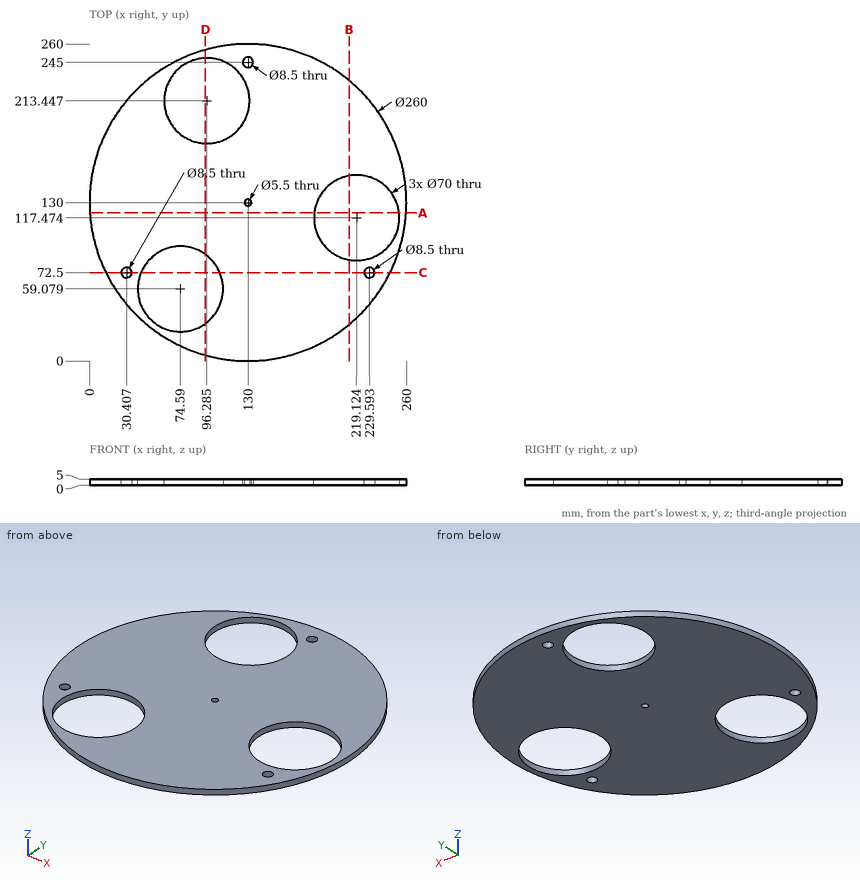
Drawing for the job (mm, zero at the part's lowest x, y, z). Round coordinates to 2 decimals unless told otherwise and drop trailing zeros. Write each loop counter-clockwise with the first axis right and the second up, starting at its lowest first coordinate (ties: lowest second). Pieces come first, ordered by that corner, then holes. Notation, with made-up numbers: M 66.5,-14.5 L 108.5,-14.5 A18 cw 108.5,-9.5 Z; hole C 5.5,47 d8. An arc over 180 degrees is marked long. Answer in a Markdown table with one row per item.
1. Saw through at A-A (y = 121.5). List the corners of the cut face in (x, z).
Geometry check:
| item | result |
|---|---|
| outline | M 0.28,0 L 184.36,0 L 184.36,5 L 0.28,5 Z; M 253.89,0 L 259.72,0 L 259.72,5 L 253.89,5 Z |
2. Saw through at D-D (x = 95). List the corners of the cut face in (y, z) (1 decimal).
Geometry check:
| item | result |
|---|---|
| outline | M 4.8,0 L 30.6,0 L 30.6,5 L 4.8,5 Z; M 87.5,0 L 178.5,0 L 178.5,5 L 87.5,5 Z; M 248.4,0 L 255.2,0 L 255.2,5 L 248.4,5 Z |
3. Probe L1, parallel to Y at x = 97, z = 2.85 (1 decimal); L2, parallel to X at y = 128, z = 2.9 (1 decimal); L3, parallel to Y at x = 69, z = 4.7 (1 decimal). List the from-to ranges inside material, lowest first. Write a range as [from, to].
Geometry check:
| item | result |
|---|---|
| L1 | [4.3, 32.2], [86, 178.5], [248.4, 255.7] |
| L2 | [0, 128.1], [131.9, 185.7], [252.5, 260] |
| L3 | [15.2, 24.5], [93.6, 191.5], [235.4, 244.8] |
4. Flat gauge pins, fed straight in: P1, Ø13.5, axis at x = 229.59, y = 72.5, coming from the -Z side; P2, Ø1.5, axis at x = 28.5, z = 4, coming from the -Y side (1 decimal); P3, Ø1, axis at x = 58, z = 1.5, coming from the +Y side; P4, Ø1, axis at y = 134.5, z = 1.5, coming from the -X side. Where does each tip first touch, or does it go through?
Geometry check:
| item | result |
|---|---|
| P1 | z = 0 |
| P2 | y = 47.8 |
| P3 | y = 238.57 |
| P4 | x = 0.06 |
5. Saw through at C-C (y = 72.5). List the corners of the cut face in (x, z) (1 decimal).
Geometry check:
| item | result |
|---|---|
| outline | M 13.4,0 L 26.2,0 L 26.2,5 L 13.4,5 Z; M 34.7,0 L 42.3,0 L 42.3,5 L 34.7,5 Z; M 106.9,0 L 225.3,0 L 225.3,5 L 106.9,5 Z; M 233.8,0 L 246.6,0 L 246.6,5 L 233.8,5 Z |
6. Saw through at B-B (x = 213). List the corners of the cut face in (y, z) (1 decimal).
Geometry check:
| item | result |
|---|---|
| outline | M 29.9,0 L 83,0 L 83,5 L 29.9,5 Z; M 151.9,0 L 230.1,0 L 230.1,5 L 151.9,5 Z |
